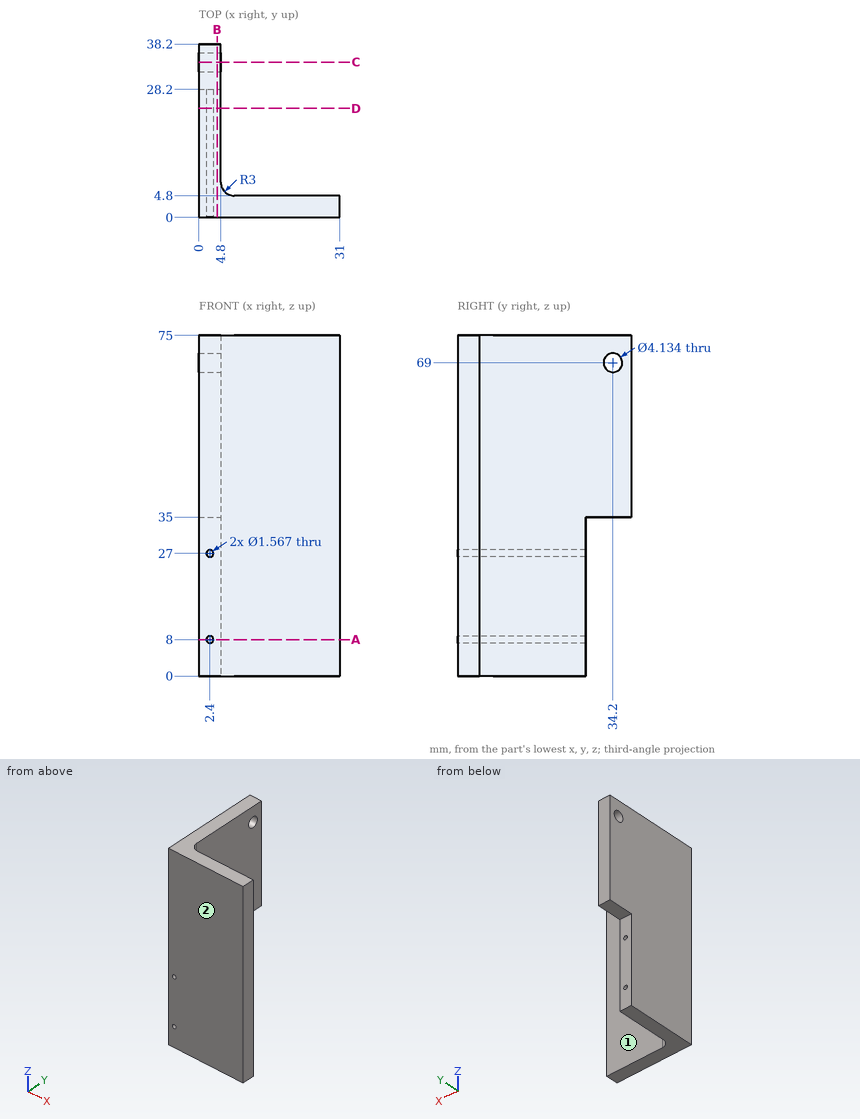
Source: three-view drawing plus pictorial views. Frame: mm from the lowest corner of the part. A direction names the side the tool comes from. Give positions to 0.01 mm unless a question says otherwise; leave off trailing zeros. Order: outer loops, then holes, each group sorted by start corner. A loop starts at its lowest first (then second) coordinate and runs counter-clockwise, first axis right, second up. Notation, with made-up numbers: (79, 86.25) - (118, 86.25) arc R27 ccw to (118, 117.25) - close; hole circle Ø9 at (74.25, -29). An arc over 180 degrees is marked (long way). Answer as a JSON object with one key per item and string values. Group by question number.
Q1. Cut plane A-A, the plane z = 8. Output: boundary loops of the cut face in (x, y).
Q2. Cut plane B-B, the plane x = 4. Output: boundary loops of the cut face in (y, z), then the cut area to 3 significant figures.
Q3. First-contact query: pin 1 Ø8 at (x, y) = (15, 11) entering from +Z; pin 2 Ø1.4 at (x, z) = (1.5, 12.5) entering from +Y; pin 3 Ø18.5 at (x, z) = (24, 49.5) entering from +Y; pin 4 Ø1.4 at (x, y) = (2, 33) entering from -Z. Flat tips, straight axial feed; report the tip coordinate or a pass-through.
Q4. Line query: probe 1 along Z at (x, y) = (2.4, 11.5); probe 2 along Y at (x, z) = (3.1, 69); probe 3 along X at (y, z) = (10.75, 27). Output: solid intervals per line, ascending.
Q5. Cut plane D-D, the plane y = 24. Output: boundary loops of the cut face in (x, z), then the cut area to 3 significant figures.
Q6. Set-up query: the marked faces 1 and 2. Return all of +Z, -Z, +X, -X, +Y, -Y with unobstructed straight access to the full face (end or side cutting, diameter ignored); none if empty.
Q7. Cut plane C-C, the plane y = 34.2. Output: boundary loops of the cut face in (x, z).
Results:
{
 "1": {"outline": "(0, 0) - (1.62, 0) - (1.62, 28.2) - (0, 28.2) - close; (3.18, 0) - (31, 0) - (31, 4.8) - (7.8, 4.8) arc R3 cw to (4.8, 7.8) - (4.8, 28.2) - (3.18, 28.2) - close"},
 "2": {"outline": "(0, 0) - (28.2, 0) - (28.2, 35) - (38.2, 35) - (38.2, 75) - (0, 75) - close; hole circle Ø4.13 at (34.2, 69)", "area": "2,500 mm^2"},
 "3": {"pin 1": "through", "pin 2": "y = 28.2", "pin 3": "y = 4.8", "pin 4": "z = 35"},
 "4": {"probe 1": "0 to 7.22, 8.78 to 26.22, 27.78 to 75", "probe 2": "0 to 32.13, 36.27 to 38.2", "probe 3": "0 to 1.62, 3.18 to 4.8"},
 "5": {"outline": "(0, 0) - (4.8, 0) - (4.8, 75) - (0, 75) - close; hole circle Ø1.57 at (2.4, 8); hole circle Ø1.57 at (2.4, 27)", "area": "356 mm^2"},
 "6": {"face 1": "+Z, -Z, +X, +Y", "face 2": "+Z, -Z, +X, -X, -Y"},
 "7": {"outline": "(0, 35) - (4.8, 35) - (4.8, 66.93) - (0, 66.93) - close; (0, 71.07) - (4.8, 71.07) - (4.8, 75) - (0, 75) - close"}
}
